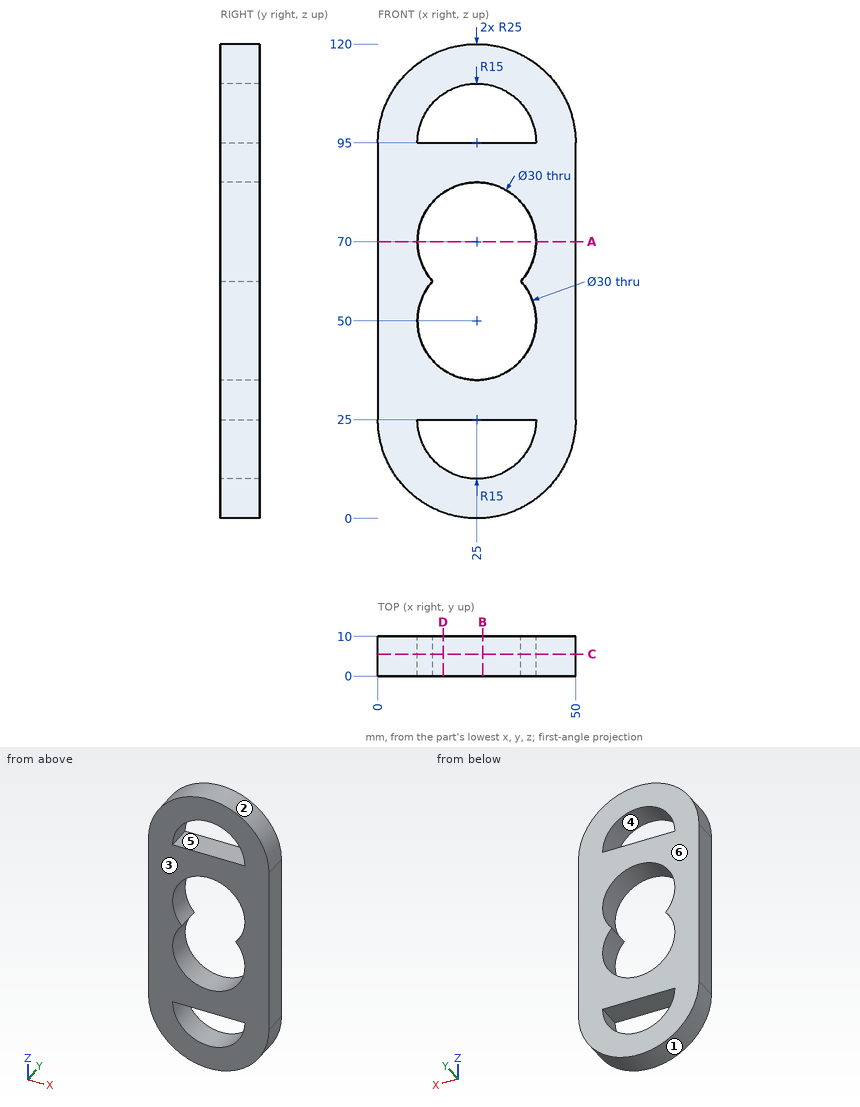
Check sheet for the drawn part. Datum: minimum x, y, z corner. Units: mm. A direction names the side the tool comes from. Give positions to 0.01 mm unless a question says otherwise; leave off trailing zeros. Loops run counter-clockwise (first coordinate to the right, second up) from the corner with the lowest first, then second, coordinate; pieces in that order, holes last. Notation, with made-up numbers: M 28.25,54.25 L 75.25,54.25 A18 ccw 75.25,59.25 Z; hole C 15,-5 d6. An arc over 180 degrees is marked long. Return JSON: item names as keys, results as strings.
1) Section check A-A, the plane z = 70. Enter the section's corners in (x, y), and give its area (3 significant figures).
Findings:
{"outline": "M 0,0 L 10,0 L 10,10 L 0,10 Z; M 40,0 L 50,0 L 50,10 L 40,10 Z", "area": "200 mm2"}
2) Section check C-C, the plane y = 5.5. Enter the section's corners in (x, z), and give its area (3 significant figures).
Findings:
{"outline": "M 0,25 A25 ccw 50,25 L 50,95 A25 ccw 0,95 Z; hole M 10,25 A15 ccw 40,25 Z; hole M 10,95 L 40,95 A15 ccw Z; hole M 13.82,60 A15 ccw long 36.18,60 A15 ccw long Z", "area": "3,500 mm2"}
3) Section check D-D, the plane x = 16.5. Enter the section's corners in (y, z).
Findings:
{"outline": "M 0,1.49 L 10,1.49 L 10,12.64 L 0,12.64 Z; M 0,25 L 10,25 L 10,37.64 L 0,37.64 Z; M 0,82.36 L 10,82.36 L 10,95 L 0,95 Z; M 0,107.36 L 10,107.36 L 10,118.51 L 0,118.51 Z"}
4) Mould release check, pull along Z, two halves, no side actions. Record for the marked faces 1, 2, 3 and 4: released by +Z, released by -Z, zero draft, split by the parting line, or undercut.
Findings:
{"face 1": "released by -Z", "face 2": "released by +Z", "face 3": "zero draft", "face 4": "undercut"}
5) Tool access check on the marked faces 5 and 6. Record the directions out of +Z, -Z, +X, -X, +Y, -Y that give a thin tool (end or side, any length) a straight path to the whole face; none if there is none.
Findings:
{"face 5": "+Y, -Y", "face 6": "+Z, -Z, +X, -X, +Y"}
6) Gauge pin test, flat ends, axial feed: P1, Ø1, axis at x = 16, y = 7, coming from the -Z side; P2, Ø3, axis at x = 25.5, y = 4, coming from the +Z side; P3, Ø1.5, axis at x = 19, z = 81.5, coming from the +Y side; P4, Ø5, axis at x = 42.5, y = 8, coming from the +Z side. Record the tip position at first contact, or that the pin passes through.
Findings:
{"P1": "stops at z = 1.49", "P2": "stops at z = 120", "P3": "passes through", "P4": "stops at z = 115"}
7) Section check B-B, the plane x = 26.5. Enter the section's corners in (y, z), and give its area (3 significant figures).
Findings:
{"outline": "M 0,0.05 L 10,0.05 L 10,10.08 L 0,10.08 Z; M 0,25 L 10,25 L 10,35.08 L 0,35.08 Z; M 0,84.92 L 10,84.92 L 10,95 L 0,95 Z; M 0,109.92 L 10,109.92 L 10,119.95 L 0,119.95 Z", "area": "402 mm2"}
8) Material ranges on L1, parallel to Z at x = 25, y = 4.5; L2, parallel to X at y = 6.75, z = 50; L3, parallel to Z at x = 38, y = 5.5, recorded low to high. Write a range as [from, to].
Findings:
{"L1": "z = [0, 10], [25, 35], [85, 95], [110, 120]", "L2": "x = [0, 10], [40, 50]", "L3": "z = [3.65, 17.52], [25, 42.52], [57.48, 62.52], [77.48, 95], [102.48, 116.35]"}
